Part model, mm, in its own coordinate system. A direction names the side the tool comes from. Give positions to 0.01 mm unless a question says otherwise; leave off trailing zeros. Order: outer loops, then holes, each group sorted by start corner. A loop starts at its lowest first (then second) coordinate and runs counter-clockwise, first axis right, second up.
1. Drop flat-ended pins along their axis: pin 1 Ø10 at (x, z) = (-11, 7.5) entering from +Y; pin 2 Ø6.5 at (x, z) = (0, 0) entering from -Y; pin 3 Ø4 at (x, z) = (0, 9.5) entering from -Y. Give the stop position or say it passes through.
2. Slice it at C-C on y = 20.5. List the corners of the cut face in (x, z), and give its area (3 significant figures).
3. Slice it at B-B on x = 0. List the corners of the cut face in (y, z).
4. Probe line 1 (Z direction, x = 0, y = 2.75); line 2 (Z direction, x = 0, y = 3.1); line 3 (Z direction, x = 0, y = 1.4). List the from-to ranges inside material, lowest first.
5. Slice it at A-A on z = 0. List the corners of the cut face in (x, y).
6. Which spindle directions (+Z, -Z, +X, -X, +Y, -Y) get a long thin tool onto all of the face, cutting with end or side? Do faces 4 (the cylindrical face through (-0.34, 34.93, 1.55)), 5 (the cylindrical face through (-0.54, 1.97, -11.94)), 6 (the cylindrical face through (13.21, 13.72, -4.16)). Say none if no direction does.
7. Mould opens along Z. For faces 1 (the conical face through (-2.799, 0.355, 12.606)), 2 (the flat face through (-3, 0, 3)), 3 (the cylindrical face through (-10.5, 2, 0.1)) say: +Z half, -Z half, draft (parallel to the pull), parting line (faces both ways), or undercut.
from build123d import *

# Parameters (mm, degrees)
CROQUIS1_R              = 13.85
SALIENTE_EXTRUIR1_DEPTH = 26
CHAFL_N1_SIZE           = 1
CHAFL_N1_SIZE2          = 5.67128182
CHAFL_N2_SIZE           = 4
CROQUIS3_R              = 5
SALIENTE_EXTRUIR3_DEPTH = 4
CROQUIS4_R              = 1.5875
SALIENTE_EXTRUIR4_DEPTH = 10
CROQUIS5_R              = 2.5
CORTAR_EXTRUIR1_DEPTH   = 4
CROQUIS6_R              = 4
CORTAR_EXTRUIR2_DEPTH   = 1.5


with BuildPart() as part:
    # Croquis1 → Saliente-Extruir1 (new body)
    with BuildSketch(Plane(origin=(0, 0, 0), x_dir=(1, 0, 0), z_dir=(0, 1, 0))):
        Circle(CROQUIS1_R)
    extrude(amount=SALIENTE_EXTRUIR1_DEPTH)

    # Chaflán1
    chafl_n1_edges = [part.edges().sort_by_distance(p)[0] for p in [
        (-13.85, 0, 0),
    ]]
    chafl_n1_side = [part.faces().sort_by_distance(p)[0] for p in [
        (0, 0, 0),
    ]]
    chamfer(chafl_n1_edges, length=CHAFL_N1_SIZE, length2=CHAFL_N1_SIZE2, reference=chafl_n1_side[0])

    # Chaflán2
    chafl_n2_edges = [part.edges().sort_by_distance(p)[0] for p in [
        (-13.85, 26, 0),
    ]]
    chamfer(chafl_n2_edges, length=CHAFL_N2_SIZE)

    # Croquis3 → Saliente-Extruir3 (add)
    with BuildSketch(Plane(origin=(0, 26, 0), x_dir=(1, 0, 0), z_dir=(0, 1, 0))):
        Circle(CROQUIS3_R)
    extrude(amount=SALIENTE_EXTRUIR3_DEPTH)

    # Croquis4 → Saliente-Extruir4 (add)
    with BuildSketch(Plane(origin=(0, 30, 0), x_dir=(1, 0, 0), z_dir=(0, 1, 0))):
        Circle(CROQUIS4_R)
    extrude(amount=SALIENTE_EXTRUIR4_DEPTH)

    # Croquis5 → Cortar-Extruir1 (cut)
    with BuildSketch(Plane.XZ):
        with Locations((8, 0)):
            Circle(CROQUIS5_R)
        with Locations((0, 9.5)):
            Circle(CROQUIS5_R)
        with Locations((0, -9.5)):
            Circle(CROQUIS5_R)
        with Locations((-8, 0)):
            Circle(CROQUIS5_R)
    extrude(amount=-CORTAR_EXTRUIR1_DEPTH, mode=Mode.SUBTRACT)

    # Croquis6 → Cortar-Extruir2 (cut)
    with BuildSketch(Plane.XZ):
        Circle(CROQUIS6_R)
    extrude(amount=-CORTAR_EXTRUIR2_DEPTH, mode=Mode.SUBTRACT)


solid = part.part
Data:
1. pin 1: stops at y = 26
1. pin 2: stops at y = 1.5
1. pin 3: stops at y = 4
2. outline: circle Ø27.7 at (0, 0)
2. area: 603 mm2
3. outline: (0, -12.85) - (5.67, -13.85) - (22, -13.85) - (26, -9.85) - (26, -5) - (30, -5) - (30, -1.59) - (40, -1.59) - (40, 1.59) - (30, 1.59) - (30, 5) - (26, 5) - (26, 9.85) - (22, 13.85) - (5.67, 13.85) - (0, 12.85) - (0, 12) - (4, 12) - (4, 7) - (0, 7) - (0, 4) - (1.5, 4) - (1.5, -4) - (0, -4) - (0, -7) - (4, -7) - (4, -12) - (0, -12) - close
4. line 1: z = -13.33 to -12, -7 to 7, 12 to 13.33
4. line 2: z = -13.4 to -12, -7 to 7, 12 to 13.4
4. line 3: z = -13.1 to -12, -7 to -4, 4 to 7, 12 to 13.1
5. outline: (-13.85, 5.67) - (-12.85, 0) - (-10.5, 0) - (-10.5, 4) - (-5.5, 4) - (-5.5, 0) - (-4, 0) - (-4, 1.5) - (4, 1.5) - (4, 0) - (5.5, 0) - (5.5, 4) - (10.5, 4) - (10.5, 0) - (12.85, 0) - (13.85, 5.67) - (13.85, 22) - (9.85, 26) - (5, 26) - (5, 30) - (1.59, 30) - (1.59, 40) - (-1.59, 40) - (-1.59, 30) - (-5, 30) - (-5, 26) - (-9.85, 26) - (-13.85, 22) - close
6. face 4: +Y
6. face 5: -Y
6. face 6: +Y, -Y
7. face 1: parting line
7. face 2: draft
7. face 3: undercut
